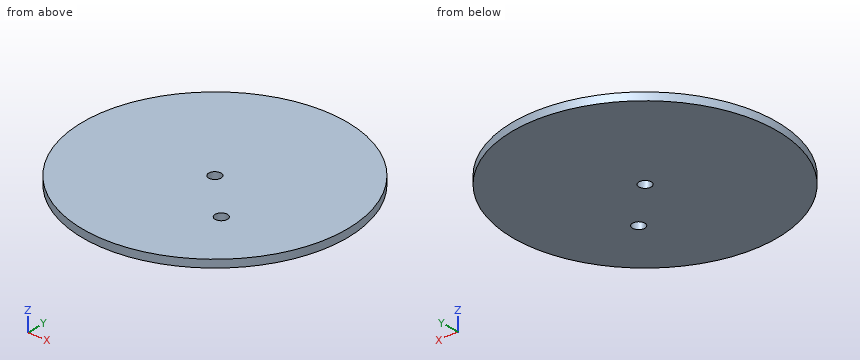
```python
from build123d import *

# Parameters (mm, degrees)
SKETCH1_R                = 42.5
SKETCH1_R_2              = 2
BOSS_EXTRUDE1_DEPTH      = 1.25
BOSS_EXTRUDE1_DEPTH_BACK = 1.25


with BuildPart() as part:
    # Sketch1 → Boss-Extrude1 (new body, two sides)
    with BuildSketch(Plane.XY) as boss_extrude1_sk:
        Circle(SKETCH1_R)
        Circle(SKETCH1_R_2, mode=Mode.SUBTRACT)
        with Locations((14.715815051, -14.981481481)):
            Circle(SKETCH1_R_2, mode=Mode.SUBTRACT)
    extrude(amount=BOSS_EXTRUDE1_DEPTH)
    extrude(boss_extrude1_sk.sketch, amount=-BOSS_EXTRUDE1_DEPTH_BACK)


solid = part.part
```
Source: CAD feature listing. Evaluate the final solid. Frame: model axes, mm. Give positions to 0.01 mm unless a question says otherwise; leave off trailing zeros. Order: outer loops, then holes, each group sorted by start corner. A loop starts at its lowest first (then second) coordinate and runs counter-clockwise, first axis right, second up.
(1) Contact query for flat-ended pins moving along their axis: P1, Ø1.5, axis at x = -29.5, z = 0.5, coming from the +Y side; P2, Ø1, axis at x = 29, z = -0.5, coming from the +Y side. Output: stop coordinate, or through.
(2) Section query A-A (x = 0). Return the cut outline in (y, z).
(3) Section query C-C (z = -0.35). Return the cut outline in (x, y), plus the area to 3 significant figures.
(4) Section query D-D (x = 23.5). Return the cut outline in (y, z), plus the area to 3 significant figures.
(5) Material intervals for line 1 along Y through (x, z) = (0, -0.1); line 2 along X through (y, z) = (23, -0.8); line 3 along X through (y, z) = (11.5, 0.3), sorted ascending.
Outcome:
1. P1: stops at y = 31.3
1. P2: stops at y = 31.53
2. outline: (-42.5, -1.25) - (-2, -1.25) - (-2, 1.25) - (-42.5, 1.25) - close; (2, -1.25) - (42.5, -1.25) - (42.5, 1.25) - (2, 1.25) - close
3. outline: circle Ø85 at (0, 0); hole circle Ø4 at (0, 0); hole circle Ø4 at (14.72, -14.98)
3. area: 5,650 mm2
4. outline: (-35.41, -1.25) - (35.41, -1.25) - (35.41, 1.25) - (-35.41, 1.25) - close
4. area: 177 mm2
5. line 1: y = -42.5 to -2, 2 to 42.5
5. line 2: x = -35.74 to 35.74
5. line 3: x = -40.91 to 40.91
